Geometry: final body of the model. Coordinates: model frame, mm. A direction names the side the tool comes from. Give positions to 0.01 mm unless a question says otherwise; leave off trailing zeros. Order: outer loops, then holes, each group sorted by start corner. A loop starts at its lowest first (then second) coordinate and runs counter-clockwise, first axis right, second up. Notation, with made-up numbers: (50.5, 33) - (68.5, 33) arc R12 cw to (68.5, 42) - close; hole circle Ø7 at (70, 59.5). An arc over 180 degrees is marked (long way). Use one line per item in the form item = value.
from build123d import *

# Parameters (mm, degrees)
BOSS_EXTRUDE1_DEPTH   = 1
SKETCH3_R             = 2.6162
BOSS_EXTRUDE1_2_DEPTH = 1
SKETCH4_R             = 2.6162
BOSS_EXTRUDE2_DEPTH   = 1.5
BOSS_EXTRUDE3_DEPTH   = 3
SKETCH6_W             = 15.9258
SKETCH6_H             = 13.25
BOSS_EXTRUDE4_DEPTH   = 5
SKETCH7_W             = 13.5128
SKETCH7_H             = 10
CUT_EXTRUDE1_DEPTH    = 5
FILLET1_R             = 2.54
FILLET2_R             = 2.54
FILLET3_R             = 7.62
FILLET5_R             = 2.54
SKETCH8_W             = 15.9258
SKETCH8_H             = 10.5
CUT_EXTRUDE2_DEPTH    = 3
BOSS_EXTRUDE5_DEPTH   = 4
SKETCH10_W            = 0.6964
SKETCH10_H            = 7.5
BOSS_EXTRUDE6_DEPTH   = 2
FILLET8_R             = 2


with BuildPart() as part:
    # Sketch3 → Boss-Extrude1 (new body)
    with BuildSketch(Plane(origin=(0, 0, 0), x_dir=(1, 0, 0), z_dir=(0, 1, 0))):
        Polygon((6.7564, 24.25), (6.7564, 20.22), (7.9629, 20.22), (7.9629, 25.5), (-7.9629, 25.5), (-7.9629, 20.22), (-6.7564, 20.22), (-6.7564, 24.25), align=None)
    extrude(amount=BOSS_EXTRUDE1_DEPTH)



with BuildPart() as body_2:
    # Sketch3 → Boss-Extrude1 2 (new body)
    with BuildSketch(Plane(origin=(0, 0, 0), x_dir=(1, 0, 0), z_dir=(0, 1, 0))):
        with BuildLine():
            Line((6.7564, 12.6), (6.7564, 4.876812672))
            ThreePointArc((6.7564, 4.876812672), (6.776225919, 4.847421317), (6.796505263, 4.818340964))
            ThreePointArc((6.796505263, 4.818340964), (0, -8.3312), (-6.796505263, 4.818340964))
            ThreePointArc((-6.796505263, 4.818340964), (-6.776225919, 4.847421317), (-6.7564, 4.876812672))
            Line((-6.7564, 4.876812672), (-6.7564, 12.6))
            Line((-6.7564, 12.6), (-7.9629, 12.6))
            Line((-7.9629, 12.6), (-7.9629, 10.019330915))
            ThreePointArc((-7.9629, 10.019330915), (-8.553832276, 8.174549356), (-10.10666, 7.016470768))
            Line((-10.10666, 7.016470768), (-17.42186, 4.50429022))
            ThreePointArc((-17.42186, 4.50429022), (-20.6375, 0), (-17.42186, -4.50429022))
            Line((-17.42186, -4.50429022), (-3.22159376, -9.380935099))
            ThreePointArc((-3.22159376, -9.380935099), (0, -9.9187), (3.22159376, -9.380935099))
            Line((3.22159376, -9.380935099), (17.42186, -4.50429022))
            ThreePointArc((17.42186, -4.50429022), (20.6375, 0), (17.42186, 4.50429022))
            Line((17.42186, 4.50429022), (10.10666, 7.016470768))
            ThreePointArc((10.10666, 7.016470768), (8.553832276, 8.174549356), (7.9629, 10.019330915))
            Line((7.9629, 10.019330915), (7.9629, 12.6))
            Line((7.9629, 12.6), (6.7564, 12.6))
        make_face()
        with Locations(Location((-15.875, 0, 0), (0, 0, 270))):
            Circle(SKETCH3_R, mode=Mode.SUBTRACT)
        with Locations(Location((15.875, 0, 0), (0, 0, 270))):
            Circle(SKETCH3_R, mode=Mode.SUBTRACT)
    extrude(amount=BOSS_EXTRUDE1_2_DEPTH)


with BuildPart() as part_1:
    add(part.part)

    add(body_2.part)  # Boss-Extrude2 merges body 2
    # Sketch4 → Boss-Extrude2 (add)
    with BuildSketch(Plane(origin=(0, 1, 0), x_dir=(1, 0, 0), z_dir=(0, 1, 0))):
        with BuildLine():
            Line((7.9629, 20.22), (7.9629, 25.5))
            Line((7.9629, 25.5), (-7.9629, 25.5))
            Line((-7.9629, 25.5), (-7.9629, 20.22))
            Line((-7.9629, 20.22), (-7.9629, 12.6))
            Line((-7.9629, 12.6), (-7.9629, 10.019330915))
            ThreePointArc((-7.9629, 10.019330915), (-8.553832276, 8.174549356), (-10.10666, 7.016470768))
            Line((-10.10666, 7.016470768), (-17.42186, 4.50429022))
            ThreePointArc((-17.42186, 4.50429022), (-20.6375, 0), (-17.42186, -4.50429022))
            Line((-17.42186, -4.50429022), (-3.22159376, -9.380935099))
            ThreePointArc((-3.22159376, -9.380935099), (0, -9.9187), (3.22159376, -9.380935099))
            Line((3.22159376, -9.380935099), (17.42186, -4.50429022))
            ThreePointArc((17.42186, -4.50429022), (20.6375, 0), (17.42186, 4.50429022))
            Line((17.42186, 4.50429022), (10.10666, 7.016470768))
            ThreePointArc((10.10666, 7.016470768), (8.553832276, 8.174549356), (7.9629, 10.019330915))
            Line((7.9629, 10.019330915), (7.9629, 12.6))
            Line((7.9629, 12.6), (7.9629, 20.22))
        make_face()
        with Locations(Location((15.875, 0, 0), (0, 0, 270))):
            Circle(SKETCH4_R, mode=Mode.SUBTRACT)
        with Locations(Location((-15.875, 0, 0), (0, 0, 270))):
            Circle(SKETCH4_R, mode=Mode.SUBTRACT)
        with BuildLine():
            Line((-6.7564, 24.25), (6.7564, 24.25))
            Line((6.7564, 24.25), (6.7564, 20.22))
            Line((6.7564, 20.22), (6.7564, 12.6))
            Line((6.7564, 12.6), (6.7564, 4.876812672))
            ThreePointArc((6.7564, 4.876812672), (6.776225919, 4.847421317), (6.796505263, 4.818340964))
            ThreePointArc((6.796505263, 4.818340964), (0, -8.3312), (-6.796505263, 4.818340964))
            ThreePointArc((-6.796505263, 4.818340964), (-6.776225919, 4.847421317), (-6.7564, 4.876812672))
            Line((-6.7564, 4.876812672), (-6.7564, 12.6))
            Line((-6.7564, 12.6), (-6.7564, 20.22))
            Line((-6.7564, 20.22), (-6.7564, 24.25))
        make_face(mode=Mode.SUBTRACT)
    extrude(amount=BOSS_EXTRUDE2_DEPTH)

    # Sketch5 → Boss-Extrude3 (add)
    # profile 1 of 2: a face of its own
    with BuildSketch(Plane(origin=(0, 2.5, 0), x_dir=(1, 0, 0), z_dir=(0, 1, 0))):
        with BuildLine():
            Line((-10.10666, 7.016470768), (-9.91527155, -0.260767662))
            ThreePointArc((-9.91527155, -0.260767662), (-7.996166023, -5.868725468), (-3.22159376, -9.380935099))
            ThreePointArc((-3.22159376, -9.380935099), (0, -9.9187), (3.22159376, -9.380935099))
            ThreePointArc((3.22159376, -9.380935099), (7.996166023, -5.868725468), (9.91527155, -0.260767662))
            Line((9.91527155, -0.260767662), (10.10666, 7.016470768))
            ThreePointArc((10.10666, 7.016470768), (8.553832276, 8.174549356), (7.9629, 10.019330915))
            Line((7.9629, 10.019330915), (7.9629, 25.5))
            Line((7.9629, 25.5), (-7.9629, 25.5))
            Line((-7.9629, 25.5), (-7.9629, 10.019330915))
            ThreePointArc((-7.9629, 10.019330915), (-8.553832276, 8.174549356), (-10.10666, 7.016470768))
        make_face()
        with BuildLine():
            Line((-6.7564, 4.876812672), (-6.7564, 24.25))
            Line((-6.7564, 24.25), (6.7564, 24.25))
            Line((6.7564, 24.25), (6.7564, 4.876812672))
            ThreePointArc((6.7564, 4.876812672), (6.776225919, 4.847421317), (6.796505263, 4.818340964))
            ThreePointArc((6.796505263, 4.818340964), (0, -8.3312), (-6.796505263, 4.818340964))
            ThreePointArc((-6.796505263, 4.818340964), (-6.776225919, 4.847421317), (-6.7564, 4.876812672))
        make_face(mode=Mode.SUBTRACT)
    # profile 2 of 2: a face of its own
    with BuildSketch(Plane(origin=(0, 2.5, 0), x_dir=(1, 0, 0), z_dir=(0, 1, 0))):
        with BuildLine():
            ThreePointArc((-6.796505263, 4.818340964), (-6.776225919, 4.847421317), (-6.7564, 4.876812672))
            Line((-6.7564, 4.876812672), (-6.7564, 24.25))
            Line((-6.7564, 24.25), (6.7564, 24.25))
            Line((6.7564, 24.25), (6.7564, 4.876812672))
            ThreePointArc((6.7564, 4.876812672), (6.776225919, 4.847421317), (6.796505263, 4.818340964))
            ThreePointArc((6.796505263, 4.818340964), (0, -8.3312), (-6.796505263, 4.818340964))
        make_face()
    extrude(amount=BOSS_EXTRUDE3_DEPTH)

    # Sketch6 → Boss-Extrude4 (add)
    with BuildSketch(Plane(origin=(0, 5.5, 0), x_dir=(1, 0, 0), z_dir=(0, 1, 0))):
        with Locations((0, 18.875)):
            Rectangle(SKETCH6_W, SKETCH6_H)
    extrude(amount=BOSS_EXTRUDE4_DEPTH)

    # Sketch7 → Cut-Extrude1 (cut)
    with BuildSketch(Plane.XZ.offset(-2.5)):
        with Locations((0, -19.25)):
            Rectangle(SKETCH7_W, SKETCH7_H)
    extrude(amount=-CUT_EXTRUDE1_DEPTH, mode=Mode.SUBTRACT)

    # Fillet1
    fillet1_edges = [part_1.edges().sort_by_distance(p)[0] for p in [
        (-6.7564, 1.25, -4.876812672),
    ]]
    fillet(fillet1_edges, radius=FILLET1_R)

    # Fillet2
    fillet2_edges = [part_1.edges().sort_by_distance(p)[0] for p in [
        (6.7564, 1.25, -4.876812672),
    ]]
    fillet(fillet2_edges, radius=FILLET2_R)

    # Fillet3
    fillet3_edges = [part_1.edges().sort_by_distance(p)[0] for p in [
        (10.10666, 4, -7.016470768),
        (-10.10666, 4, -7.016470768),
    ]]
    fillet(fillet3_edges, radius=FILLET3_R)

    # Fillet5
    fillet5_edges = [part_1.edges().sort_by_distance(p)[0] for p in [
        (0, 5.5, -12.25),
    ]]
    fillet(fillet5_edges, radius=FILLET5_R)

    # Sketch8 → Cut-Extrude2 (cut)
    with BuildSketch(Plane(origin=(0, 0, -25.5), x_dir=(-1, 0, 0), z_dir=(0, 0, -1))):
        with Locations((0, 5.25)):
            Rectangle(SKETCH8_W, SKETCH8_H)
    extrude(amount=-CUT_EXTRUDE2_DEPTH, mode=Mode.SUBTRACT)

    # Sketch9 → Boss-Extrude5 (add)
    with BuildSketch(Plane(origin=(0, 0, -22.5), x_dir=(-1, 0, 0), z_dir=(0, 0, -1))):
        Polygon((-6.7564, 0), (-6.7564, 7.5), (6.7564, 7.5), (6.7564, 0), (7.9629, 0), (7.9629, 10.5), (-7.9629, 10.5), (-7.9629, 0), align=None)
    extrude(amount=BOSS_EXTRUDE5_DEPTH)

    # Sketch10 → Boss-Extrude6 (add)
    with BuildSketch(Plane(origin=(0, 0, -26.5), x_dir=(-1, 0, 0), z_dir=(0, 0, -1))):
        with Locations((-6.4082, 3.75)):
            Rectangle(SKETCH10_W, SKETCH10_H)
        with Locations((6.4082, 3.75)):
            Rectangle(SKETCH10_W, SKETCH10_H)
    extrude(amount=-BOSS_EXTRUDE6_DEPTH)

    # Fillet8
    fillet8_edges = [part_1.edges().sort_by_distance(p)[0] for p in [
        (-7.9629, 5.25, -26.5),
        (7.9629, 5.25, -26.5),
    ]]
    fillet(fillet8_edges, radius=FILLET8_R)


solid = part_1.part
(1) Contact query for flat-ended pins moving along their axis: pin 1 Ø13.5 at (x, z) = (-3.5, -19) entering from -Y; pin 2 Ø1 at (x, y) = (12.5, 1.5) entering from -Z; pin 3 Ø6 at (x, z) = (-15.875, 0) entering from +Y; pin 4 Ø2.5 at (x, y) = (-3, 4) entering from -Z. Output: stop coordinate, or through.
Computed values:
pin_1 = 0
pin_2 = -6.37
pin_3 = 2.5
pin_4 = -14.25
(2) Cut plane C-C on x = 0. Output: boundary loops of the cut face in (y, z).
Computed values:
outline = (0, 8.33) - (2.5, 8.33) - (2.5, -14.25) - (7.5, -14.25) - (7.5, -26.5) - (10.5, -26.5) - (10.5, -12.25) - (8.04, -12.25) arc R2.54 cw to (5.5, -9.71) - (5.5, 9.92) - (0, 9.92) - close
(3) Ray query, line 1 along X through (y, z) = (0.65, 0); line 2 along Y through (x, z) = (14, 3); line 3 along Y through (x, z) = (-7, -16). Return the intervals inside material, ascending.
Computed values:
line_1 = -20.64 to -18.49, -13.26 to -8.33, 8.33 to 13.26, 18.49 to 20.64
line_2 = 0 to 2.5
line_3 = 1 to 10.5
(4) Cut plane A-A on z = -18.5. Output: boundary loops of the cut face in (x, y).
Computed values:
outline = (-7.96, 1) - (-6.76, 1) - (-6.76, 7.5) - (6.76, 7.5) - (6.76, 1) - (7.96, 1) - (7.96, 10.5) - (-7.96, 10.5) - close
(5) Cut plane B-B on y = 3. Output: boundary loops of the cut face in (x, z) (3 decimals).
Computed values:
outline = (-10.014, -3.485) arc R7.62 ccw to (-8.567, -8.156) arc R3.175 cw to (-7.963, -10.019) - (-7.963, -24.5) arc R2 ccw to (-6.06, -26.498) - (-6.06, -24.5) - (-6.756, -24.5) - (-6.756, -14.25) - (6.756, -14.25) - (6.756, -24.5) - (6.06, -24.5) - (6.06, -26.498) arc R2 ccw to (7.963, -24.5) - (7.963, -10.019) arc R3.175 cw to (8.567, -8.156) arc R7.62 ccw to (10.014, -3.485) - (9.915, 0.261) arc R9.919 ccw to (-9.915, 0.261) - close
(6) Cut plane D-D on z = -6.5. Output: boundary loops of the cut face in (x, y).
Computed values:
outline = (-11.61, 0) - (-6.76, 0) - (-6.76, 2.5) - (6.76, 2.5) - (6.76, 0) - (11.61, 0) - (11.61, 2.5) - (9.48, 2.5) - (9.48, 5.5) - (-9.48, 5.5) - (-9.48, 2.5) - (-11.61, 2.5) - close
(7) Reachability of faces 5 (the face through (7.4, 0.5, -20.22)), 6 (the face through (7.963, 5, -17)), 7 (the face through (10.222, 1.232, 6.977)) from +Z, -Z, +X, -X, +Y, -Y: full face, straight path, thin tool, end or side. Return the list, or none.
Computed values:
face_5 = +X, -X, -Y
face_6 = -Z, +X, +Y, -Y
face_7 = +Z, +X, +Y, -Y
(8) Pull-direction query (X, two-part tool) for faces 1 (the face through (-20.637, 1.232, -0.083)), 2 (the face through (8.34, 2.11, -8.52)), 3 (the face through (-18.43, 1.23, -0.57)), 4 (the face through (0, 5.5, 0)); classes: released by +X, released by -X, zero draft, split by the parting line, or undercut.
Computed values:
face_1 = released by -X
face_2 = released by +X
face_3 = undercut
face_4 = zero draft
